For this review, take the finished solid that the model builds, in its own axes (mm). Round coordinates to 2 decimals unless told otherwise and drop trailing zeros. Order: outer loops, then holes, each group sorted by start corner. A loop starts at its lowest first (then second) coordinate and runs counter-clockwise, first axis right, second up. Notation, with made-up numbers: (51, 22.25) - (93, 22.25) arc R17 cw to (93, 45.25) - close; hole circle Ø11 at (70, 70.25). An arc over 180 degrees is marked (long way). One line per item, written item: value.
Autodesk Inventor part; units mm, degrees
ref_plane "YZ Plane" through (0, 0, 0) normal (1, 0, 0) x (0, 1, 0)
ref_plane "XZ Plane" through (0, 0, 0) normal (0, 1, 0) x (-1, 0, 0)
ref_plane "XY Plane" through (0, 0, 0) normal (0, 0, 1) x (1, 0, 0)
sketch "Sketch1" plane through (0, 0, 0) normal (1, 0, 0) x (0, 1, 0)
  line L0 (127, 101.6) -> (0, 101.6)
  line L1 (0, 101.6) -> (0, 0)
  line L2 (0, 0) -> (127, 0)
  line L3 (127, 0) -> (127, 101.6)
  circle A0 centre (100.0125, 50.8) radius 14.2875
  circle A1 centre (100.0125, 50.8) radius 26.9875
  line L4 (123.3175, 64.4088) -> (101.6, 101.6)
  line L5 (123.3175, 37.1912) -> (101.6, 0)
  dimension "d0" = 101.6
  dimension "d1" = 127
  dimension "d2" = 12.7
  dimension "d3" = 50.8
  dimension "d5" = 28.575
  dimension "d6" = 101.6
  dimension "d7" = 101.6
extrude "Extrusion1" add sketch "Sketch1" along normal blind 2.9972 contours L4 A1 L5 L2 L1 L0 | A1
sketch "Sketch2" plane through (2.9972, 0, 0) normal (1, 0, 0) x (0, 0, -1)
  circle A0 centre (-88.9, 12.7) radius 1.7272
  line L0 (-101.6, 101.6) -> (-101.6, 0)
  line L1 (-101.6, 0) -> (0, 0)
  dimension "d10" = 12.7
  dimension "d11" = 12.7
  dimension "d12" = 3.4544
extrude "Extrusion2" cut sketch "Sketch2" against normal blind 2.9972
pattern_linear "Rectangular Pattern1" count 4 spacing 25.4 along (0, 0, -1) of "Extrusion2"
properties part number "Jeep Plate 2.1" material "Polycarbonate, Clear"
Item 1: Wall thickness on line 1 (Y direction, x = 1.65, z = 38.1) (3 decimals); line 2 (Z direction, x = 1.4, y = 99.5); line 3 (Z direction, x = 0.4, y = 89): over which ranges is each line inside the solid? List them lowest first.
Returned:
line 1: 0 to 10.973, 14.427 to 93.467, 106.558 to 123.825
line 2: 0 to 36.52, 65.08 to 101.6
line 3: 0 to 41.7, 59.9 to 101.6
Item 2: Take a section at C-C (y = 99.5). Write out the cut boundary in (x, z).
Returned:
outline: (0, 0) - (3, 0) - (3, 36.52) - (0, 36.52) - close; (0, 65.08) - (3, 65.08) - (3, 101.6) - (0, 101.6) - close
Item 3: Take a section at D-D (z = 22.5). Write out the cut boundary in (x, y), plus the area to 3 significant figures.
Returned:
outline: (0, 0) - (3, 0) - (3, 114.74) - (0, 114.74) - close
area: 344 mm^2
Item 4: Take a section at A-A (z = 50.8). Write out the cut boundary in (x, y) (3 decimals).
Returned:
outline: (0, 0) - (2.997, 0) - (2.997, 85.725) - (0, 85.725) - close; (0, 114.3) - (2.997, 114.3) - (2.997, 127) - (0, 127) - close
Item 5: The part is to be moulded in two halves that separate along Z. For faces 1 (the cylindrical face through (1, 127, 51)), 2 (the cylindrical face through (1.52, 12.776, 39.826)), 3 (the flat face through (1.478, 112.611, 18.856)), say which applies: +Z half, -Z half, draft (parallel to the pull), parting line (faces both ways), or undercut.
Returned:
face 1: parting line
face 2: undercut
face 3: -Z half
Item 6: Take a section at B-B (x = 0.5). Write out the cut boundary in (y, z) (1 decimal).
Returned:
outline: (0, 0) - (101.6, 0) - (123.3, 37.2) arc R27 ccw to (123.3, 64.4) - (101.6, 101.6) - (0, 101.6) - close; hole circle Ø3.5 at (12.7, 12.7); hole circle Ø3.5 at (12.7, 38.1); hole circle Ø3.5 at (12.7, 63.5); hole circle Ø3.5 at (12.7, 88.9); hole circle Ø28.6 at (100, 50.8)
Item 7: For P1, Ø1.5, axis at x = 2, z = 17.5, coming from the +Y side, flat-tipped, find the tip position at first contact; note if it passes through.
Returned:
P1: y = 112.26
